Autodesk Inventor part; units mm, degrees
ref_plane "YZ Plane" through (0, 0, 0) normal (1, 0, 0) x (0, 1, 0)
ref_plane "XZ Plane" through (0, 0, 0) normal (0, 1, 0) x (-1, 0, 0)
ref_plane "XY Plane" through (0, 0, 0) normal (0, 0, 1) x (1, 0, 0)
sketch "Sketch1" plane through (0, 0, 0) normal (0, 1, 0) x (-1, 0, 0)
  line L0 (0, 0) -> (0, -50.8)
  line L1 (0, -50.8) -> (-50.8, -50.8)
  line L2 (-50.8, -50.8) -> (-50.8, -44.45)
  line L3 (-50.8, -44.45) -> (-6.35, -44.45)
  line L4 (-6.35, -44.45) -> (-6.35, 0)
  line L5 (-6.35, 0) -> (0, 0)
  dimension "d0" = 6.35
  dimension "d1" = 50.8
extrude "Extrusion1" add sketch "Sketch1" along normal blind 152.4
sketch "Sketch2" plane through (0, 0, -50.8) normal (-1, 0, 0) x (0, 0, 1)
  point P0 (50.8, 0)
sketch "Sketch3" plane through (6.35, 0, 0) normal (1, 0, 0) x (0, 0, -1)
  line L0 (0, 0) -> (50.8, 0)
  line L1 (44.45, 0) -> (44.45, 152.4)
  line L2 (0, 0) -> (44.45, 0)
  line L3 (44.45, 0) -> (44.45, 38.1)
  line L4 (44.45, 38.1) -> (0, 38.1)
  line L5 (0, 38.1) -> (0, 0)
  dimension "d5" = 38.1
extrude "Extrusion2" cut sketch "Sketch3" against normal through all
sketch "Sketch4" plane through (6.35, 152.4, 0) normal (1, 0, 0) x (0, 0, -1)
  line L0 (0, -114.3) -> (0, 0)
  line L1 (50.8, 0) -> (0, 0)
  line L2 (0, -114.3) -> (25.4, -114.3)
  line L3 (25.4, -114.3) -> (25.4, 0)
  line L4 (25.4, 0) -> (0, 0)
  line L5 (0, 0) -> (0, -114.3)
  point P0 (0, -152.4)
  dimension "d8" = 25.4
extrude "Extrusion3" cut sketch "Sketch4" against normal through all
sketch "Sketch6" plane through (50.8, 0, -50.8) normal (0, 0, -1) x (-1, 0, 0)
  line L0 (0, 152.4) -> (50.8, 152.4)
  line L1 (0, 0) -> (0, 152.4)
  point P0 (50.8, 0)
  point P1 (22.225, 127)
  dimension "d11" = 25.4
  dimension "d12" = 22.225
hole "Hole1" at (28.575, 127, -50.8) direction (0, 0, 1) diameter 10.0838 end through all
properties part number "LiftAngleBracketExtensionLeft" material "Aluminum 6061"
Model file for the job. Use its own axes, mm. A direction names the side the tool comes from. Round coordinates to 2 decimals unless told otherwise and drop trailing zeros. Write each loop counter-clockwise with the first axis right and the second up, starting at its lowest first coordinate (ties: lowest second). Pieces come first, ordered by that corner, then holes. Notation, with made-up numbers: M 20,66.25 L 41,66.25 A20 ccw 41,100.25 Z; hole C -2,69 d11. An arc over 180 degrees is marked long. Put each result on its own line as item: value.
Item 1: Cut at B-B (z = -42). List the corners of the cut face in (x, y).
Responses:
outline: M 0,38.1 L 6.35,38.1 L 6.35,152.4 L 0,152.4 Z
Item 2: Flat gauge pins, fed straight in: P1, Ø4, axis at x = 17, y = 127.5, coming from the +Z side; P2, Ø12, axis at y = 38, z = -44, coming from the -X side; P3, Ø3, axis at x = 4.5, z = -36, coming from the -Y side; P4, Ø12, axis at y = 114, z = -35.5, coming from the +X side. Where does each tip first touch, or does it go through?
Responses:
P1: z = -44.45
P2: x = 0
P3: y = 38.1
P4: x = 6.35
Item 3: Probe L1, parallel to X at y = 127, z = -49; L2, parallel to Z at x = 26, y = 60; L3, parallel to X at y = 117, z = -44. List the from-to ranges inside material, lowest first. Write a range as from..to.
Responses:
L1: 0..23.53, 33.62..50.8
L2: -50.8..-44.45
L3: 0..6.35
Item 4: Tool access for faces 4 (the flat face through (26, 0, -48)), 5 (the flat face through (3, 38.1, -35)), 6 (the flat face through (6.35, 94, -35)): list every direction of +Z, -Z, +X, -X, +Y, -Y with a clear straight run to the whole face (end or side of a thin tool).
Responses:
face 4: +Z, -Z, +X, -X, -Y
face 5: +Z, +X, -X, -Y
face 6: +Z, +X, +Y, -Y
Item 5: Cut at C-C (y = 62). List the corners of the cut face in (x, z), and give its area (3 significant figures).
Responses:
outline: M 0,-50.8 L 50.8,-50.8 L 50.8,-44.45 L 6.35,-44.45 L 6.35,-25.4 L 0,-25.4 Z
area: 444 mm²
Item 6: Cut at A-A (y = 127). List the corners of the cut face in (x, z).
Responses:
outline: M 0,-50.8 L 23.53,-50.8 L 23.53,-44.45 L 6.35,-44.45 L 6.35,-25.4 L 0,-25.4 Z; M 33.62,-50.8 L 50.8,-50.8 L 50.8,-44.45 L 33.62,-44.45 Z
Item 7: Cut at D-D (y = 14). List the corners of the cut face in (x, z).
Responses:
outline: M 0,-50.8 L 50.8,-50.8 L 50.8,-44.45 L 0,-44.45 Z
Item 8: Mould opens along X. For faces 1 (the cylindrical face through (27.06, 131.81, -47.58)), 2 (the flat face through (26, 75, -44.45)), 3 (the flat face through (0, 92, -38)) say: +X half, -X half, draft (parallel to the pull), parting line (faces both ways), or undercut.
Responses:
face 1: undercut
face 2: draft
face 3: -X half
